Verification items for the finished model (mm, model axes). A direction names the side the tool comes from. Give positions to 0.01 mm unless a question says otherwise; leave off trailing zeros. Loops run counter-clockwise (first coordinate to the right, second up) from the corner with the lowest first, then second, coordinate; pieces in that order, holes last. Notation, with made-up numbers: (-2.75, 25.5) -> (56.25, 25.5) arc R16 ccw to (56.25, 46.5) -> close; hole circle Ø4 at (2, -23). An arc over 180 degrees is marked (long way). Answer in a Markdown table with one row per item. Add a question column.
Q1. Gauge pin test, flat ends, axial feed: P1, Ø2.5, axis at x = -6.5, y = 5.5, coming from the -Z side; P2, Ø3, axis at y = 8, z = -1, coming from the -X side (3 decimals); P3, Ø4, axis at x = 1, z = 5, coming from the +Y side. Record the tip position at first contact, or that the pin passes through.
Q2. Section check A-A on x = -9. Enter the section's corners in (y, z), and give its area (3 significant figures).
Q3. Material ranges on probe 1 along Y at (x, z) = (-9, 6.45); probe 2 along X at (y, z) = (2.5, 5.75); probe 3 along X at (y, z) = (4.25, -0.25) (3 decimals), recorded low to high.
Q4. Section check D-D on y = 2.25. Enter the section's corners in (x, z) (3 decimals).
Q5. Release check for a two-part mould opening along X. For faces 1 (the face through (-3.405, 8, 0)), 2 (the face through (-11.276, 6.777, 5.116)), 3 (the face through (12, 4, 5)), 4 (the face through (0, 8, -2.54)) record: pulls with the +X half, pulls with the -X half, needs draft (parallel to the pull), parting line crosses it, or undercut.
Q6. Section check C-C on z = -0.5. Enter the section's corners in (x, y) (3 decimals), and give its area (3 significant figures).
Q7. Section check B-B on y = 11.5. Enter the section's corners in (x, z) (3 decimals).
Q8. Set-up check for faces 5 (the face through (0, 7.541, 6)), 6 (the face through (0, 13, 2.54)), 7 (the face through (0, 4, 7.62)), 8 (the face through (7, 4, 2.54)), 9 (the face through (3.405, 8, 0)): record each of +Z, -Z, +X, -X, +Y, -Y from which the full face is reachable in a straight line by a thin tool's end or side.
```python
from build123d import *

# Parameters (mm, degrees)
SKETCH1_W           = 8.89
SKETCH1_H           = 5.08
BOSS_EXTRUDE1_DEPTH = 16.08
SKETCH2_W           = 24
SKETCH2_H           = 7.540516724
BOSS_EXTRUDE2_DEPTH = 5.08
SKETCH3_R           = 1.5
CUT_EXTRUDE1_DEPTH  = 11.16
SKETCH4_W           = 6.81
SKETCH4_H           = 3
CUT_EXTRUDE2_DEPTH  = 17.08
FILLET1_R           = 2.54


with BuildPart() as part:
    # Sketch1 → Boss-Extrude1 (new body)
    with BuildSketch(Plane(origin=(0, 0, 0), x_dir=(1, 0, 0), z_dir=(0, 1, 0))):
        Rectangle(SKETCH1_W, SKETCH1_H)
    extrude(amount=BOSS_EXTRUDE1_DEPTH)

    # Sketch2 → Boss-Extrude2 (add)
    with BuildSketch(Plane.XY.offset(2.54)):
        with Locations((0, 3.770258362)):
            Rectangle(SKETCH2_W, SKETCH2_H)
    extrude(amount=BOSS_EXTRUDE2_DEPTH)

    # Sketch3 → Cut-Extrude1 (cut, through all)
    with BuildSketch(Plane.XY.offset(7.62)):
        with Locations((-9, 3.07594)):
            Circle(SKETCH3_R)
        with Locations((9, 3.07594)):
            Circle(SKETCH3_R)
    extrude(amount=-CUT_EXTRUDE1_DEPTH, mode=Mode.SUBTRACT)

    # Sketch4 → Cut-Extrude2 (cut, through all)
    with BuildSketch(Plane(origin=(0, 16.08, 0), x_dir=(1, 0, 0), z_dir=(0, 1, 0))):
        Rectangle(SKETCH4_W, SKETCH4_H)
    extrude(amount=-CUT_EXTRUDE2_DEPTH, mode=Mode.SUBTRACT)

    # Fillet1
    fillet1_edges = [part.edges().sort_by_distance(p)[0] for p in [
        (12, 0, 5.08),
        (-12, 0, 5.08),
        (0, 7.540516724, 2.54),
        (12, 7.540516724, 5.08),
        (-12, 7.540516724, 5.08),
    ]]
    fillet(fillet1_edges, radius=FILLET1_R)


solid = part.part
```
Taken from the geometry:
| question | item | result |
|---|---|---|
| 1 | P1 | stops at z = 2.54 |
| 1 | P2 | stops at x = -4.445 |
| 1 | P3 | stops at y = 8.62 |
| 2 | outline | (0, 2.54) -> (1.58, 2.54) -> (1.58, 7.62) -> (0, 7.62) -> close; (4.58, 2.54) -> (7.54, 2.54) -> (7.54, 7.62) -> (4.58, 7.62) -> close |
| 2 | area | 23.1 mm² |
| 3 | probe 1 | y = 0 to 1.58, 4.58 to 7.54 |
| 3 | probe 2 | x = -12 to -10.39, -7.61 to 7.61, 10.39 to 12 |
| 3 | probe 3 | x = -4.445 to -3.405, 3.405 to 4.445 |
| 4 | outline | (-11.983, 2.54) -> (-10.252, 2.54) -> (-10.252, 7.62) -> (-11.983, 7.62) -> close; (-7.748, 2.54) -> (-4.445, 2.54) -> (-4.445, -2.54) -> (4.445, -2.54) -> (4.445, 2.54) -> (7.748, 2.54) -> (7.748, 7.62) -> (-7.748, 7.62) -> close; (10.252, 2.54) -> (11.983, 2.54) -> (11.983, 7.62) -> (10.252, 7.62) -> close; hole (-3.405, -1.5) -> (3.405, -1.5) -> (3.405, 1.5) -> (-3.405, 1.5) -> close |
| 5 | face 1 | undercut |
| 5 | face 2 | pulls with the -X half |
| 5 | face 3 | pulls with the +X half |
| 5 | face 4 | needs draft |
| 6 | outline | (-4.445, 0) -> (-3.405, 0) -> (-3.405, 16.08) -> (-4.445, 16.08) -> close; (3.405, 0) -> (4.445, 0) -> (4.445, 16.08) -> (3.405, 16.08) -> close |
| 6 | area | 33.4 mm² |
| 7 | outline | (-4.445, -2.54) -> (4.445, -2.54) -> (4.445, 2.54) -> (-4.445, 2.54) -> close; hole (-3.405, -1.5) -> (3.405, -1.5) -> (3.405, 1.5) -> (-3.405, 1.5) -> close |
| 8 | face 5 | +Z, +Y |
| 8 | face 6 | +Z, +X, -X, +Y |
| 8 | face 7 | +Z, +X, -X, +Y, -Y |
| 8 | face 8 | -Z, +X, +Y, -Y |
| 8 | face 9 | +Y, -Y |
